Could you check a few things on this model? Use its own coordinates, in mm. Face numbers are marked on the shaded views. A direction names the side the tool comes from. Round coordinates to 2 decimals unless told otherwise and drop trailing zeros. Write each loop counter-clockwise with the first axis right and the second up, starting at its lowest first coordinate (ties: lowest second). Pieces come first, ordered by that corner, then holes. Notation, with made-up numbers: (56.5, 26) -> (115.5, 26) arc R15 cw to (115.5, 35) -> close; hole circle Ø9 at (-32.5, 30). An arc over 180 degrees is marked (long way). Return JSON: item names as keys, results as strings.
from build123d import *

# Parameters (mm, degrees)
F0_R      = 1.6
F1_DEPTH  = 1.7
F2_W      = 50
F2_H      = 86
F3_DEPTH  = 5.4
F4_W      = 50
F4_H      = 69
F5_DEPTH  = 4
F6_W      = 46
F6_H      = 60
F7_DEPTH  = 0.1
F8_R      = 1.6
F9_DEPTH  = 1.6
F10_W     = 37
F10_H     = 18
F11_DEPTH = 11
F12_W     = 8.9
F12_H     = 14
F13_DEPTH = 10.8


with BuildPart() as f1:
    # F0 (on Top) → F1 (new body)
    with BuildSketch(Plane.XY):
        with BuildLine():
            ThreePointArc((0, 5), (1.464466, 1.464466), (5, 0))
            Line((5, 0), (145, 0))
            ThreePointArc((145, 0), (148.535534, 1.464466), (150, 5))
            Line((150, 5), (150, 95))
            ThreePointArc((150, 95), (148.535534, 98.535534), (145, 100))
            Line((145, 100), (5, 100))
            ThreePointArc((5, 100), (1.464466, 98.535534), (0, 95))
            Line((0, 95), (0, 5))
        make_face()
        with Locations((5, 5)):
            Circle(F0_R, mode=Mode.SUBTRACT)
        with Locations((65, 5)):
            Circle(F0_R, mode=Mode.SUBTRACT)
        with Locations((145, 5)):
            Circle(F0_R, mode=Mode.SUBTRACT)
        with Locations((5, 95)):
            Circle(F0_R, mode=Mode.SUBTRACT)
        with Locations((85, 95)):
            Circle(F0_R, mode=Mode.SUBTRACT)
        with Locations((145, 95)):
            Circle(F0_R, mode=Mode.SUBTRACT)
    extrude(amount=F1_DEPTH)

    # F2 (on face) → F3 (join)
    with BuildSketch(Plane.XY.offset(1.7)):
        with Locations((95, 48)):
            Rectangle(F2_W, F2_H)
    extrude(amount=F3_DEPTH)

    # F4 (on face) → F5 (join)
    with BuildSketch(Plane.XY.offset(7.1)):
        with Locations((95, 50.5)):
            Rectangle(F4_W, F4_H)
    extrude(amount=F5_DEPTH)

    # F6 (on face) → F7 (cut)
    with BuildSketch(Plane.XY.offset(11.1)):
        with Locations((95, 53)):
            Rectangle(F6_W, F6_H)
    extrude(amount=-F7_DEPTH, mode=Mode.SUBTRACT)

    # F8 (on face) → F9 (join)
    with BuildSketch(Plane.XY.offset(1.7)):
        with BuildLine():
            Line((140, 45), (140, 0))
            Line((140, 0), (160, 0))
            ThreePointArc((160, 0), (163.535534, 1.464466), (165, 5))
            Line((165, 5), (165, 40))
            ThreePointArc((165, 40), (163.535534, 43.535534), (160, 45))
            Line((160, 45), (140, 45))
        make_face()
        with Locations((145, 5)):
            Circle(F8_R, mode=Mode.SUBTRACT)
    extrude(amount=F9_DEPTH)

    # F10 (on face) → F11 (join)
    with BuildSketch(Plane(origin=(0, 0, 0), x_dir=(1, 0, 0), z_dir=(0, 0, -1))):
        with Locations((42.5, -13)):
            Rectangle(F10_W, F10_H)
    extrude(amount=F11_DEPTH)

    # F12 (on face) → F13 (join)
    with BuildSketch(Plane(origin=(0, 0, 0), x_dir=(1, 0, 0), z_dir=(0, 0, -1))):
        with Locations((132.55, -96)):
            Rectangle(F12_W, F12_H)
        with Locations((132.55, -4)):
            Rectangle(F12_W, F12_H)
    extrude(amount=F13_DEPTH)


solid = f1.part
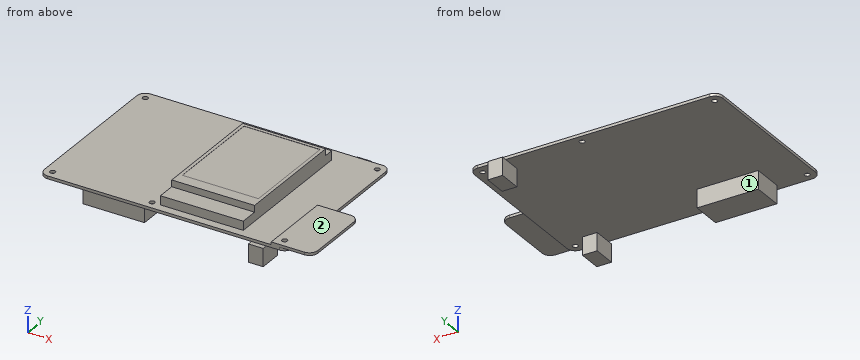
1) Will these pins go through, and if not, where does the flat tip stop? pin 1 Ø6 at (x, z) = (38.5, 1) entering from -Y; pin 2 Ø4 at (x, y) = (67.5, 34.5) entering from -Z; pin 3 Ø9 at (y, z) = (16, -5) entering from -X.
Return value:
{"pin 1": "y = 0", "pin 2": "z = 0", "pin 3": "x = 24"}
2) I want a section at A-A, the plane z = -4.5. Please give me the cut outline in (x, y).
Return value:
{"outline": "(24, 4) -> (61, 4) -> (61, 22) -> (24, 22) -> close; (128.1, -3) -> (137, -3) -> (137, 11) -> (128.1, 11) -> close; (128.1, 89) -> (137, 89) -> (137, 103) -> (128.1, 103) -> close"}
3) I want a section at D-D, the plane x = 44.5. Please give me the cut outline in (y, z).
Return value:
{"outline": "(0, 0) -> (4, 0) -> (4, -11) -> (22, -11) -> (22, 0) -> (100, 0) -> (100, 1.7) -> (0, 1.7) -> close"}
4) If I drill on probe 1 along Y at (x, z) = (145, 1.35); probe 2 along Y at (x, z) = (65, 0.45); probe 3 along X at (y, z) = (95, 0.6), over which ranges is the centre line in solid material (lowest first)? Write a range as [from, to].
Return value:
{"probe 1": "[0, 3.4], [6.6, 93.4], [96.6, 100]", "probe 2": "[0, 3.4], [6.6, 100]", "probe 3": "[0, 3.4], [6.6, 83.4], [86.6, 143.4], [146.6, 150]"}
5) I want a section at B-B, the plane x = 85. Please give me the cut outline in (y, z), and give its area (3 significant figures).
Return value:
{"outline": "(0, 0) -> (93.4, 0) -> (93.4, 1.7) -> (91, 1.7) -> (91, 7.1) -> (85, 7.1) -> (85, 11.1) -> (83, 11.1) -> (83, 11) -> (23, 11) -> (23, 11.1) -> (16, 11.1) -> (16, 7.1) -> (5, 7.1) -> (5, 1.7) -> (0, 1.7) -> close; (96.6, 0) -> (100, 0) -> (100, 1.7) -> (96.6, 1.7) -> close", "area": "899 mm²"}
6) For the marked faces 1 and 2, which set-ups out of +Z, -Z, +X, -X, +Y, -Y let a thin tool reach every point of the face, with its end or its side?
Return value:
{"face 1": "-Z, +X, -X, +Y", "face 2": "+Z, +X, +Y, -Y"}
7) I want a section at C-C, the plane y = 13.5. Please give me the cut outline in (x, z).
Return value:
{"outline": "(0, 0) -> (24, 0) -> (24, -11) -> (61, -11) -> (61, 0) -> (150, 0) -> (150, 1.7) -> (165, 1.7) -> (165, 3.3) -> (140, 3.3) -> (140, 1.7) -> (120, 1.7) -> (120, 7.1) -> (70, 7.1) -> (70, 1.7) -> (0, 1.7) -> close"}
